Geometry check sheet. Reference: the model listing, model coordinates, mm. Round coordinates to 2 decimals unless told otherwise and drop trailing zeros. Order: outer loops, then holes, each group sorted by start corner. A loop starts at its lowest first (then second) coordinate and runs counter-clockwise, first axis right, second up. Notation, with made-up numbers: (86, 46) - (143, 46) arc R14 ccw to (143, 73) - close; hole circle Ø7 at (-33, 30.25). An arc over 180 degrees is marked (long way). Use a Markdown table: item, result. Add a question column.
(1) Thickness scan on line 1 along X through (y, z) = (-140, 2.2); line 2 along Y through (x, z) = (220, 1.35); line 3 along X through (y, z) = (100.5, 2.5). Record the ranges inside material, lowest first. Write a range as [from, to].
(2) Gauge pin test, flat end, axial feed: P1, Ø3, axis at x = 260, y = -100, coming from the +Z side. Record the tip position at first contact, or that the pin passes through.
(3) Section check B-B on y = -59.5. Record the boundary of the cut face in (x, z), then the cut area to 3 significant figures.
(4) Section check C-C on x = 17.5. Record the boundary of the cut face in (y, z).
(5) Section check A-A on z = 0.8. Give the number of separate pieces and of enclosed holes in the cut face, then the cut area to 3 significant figures.
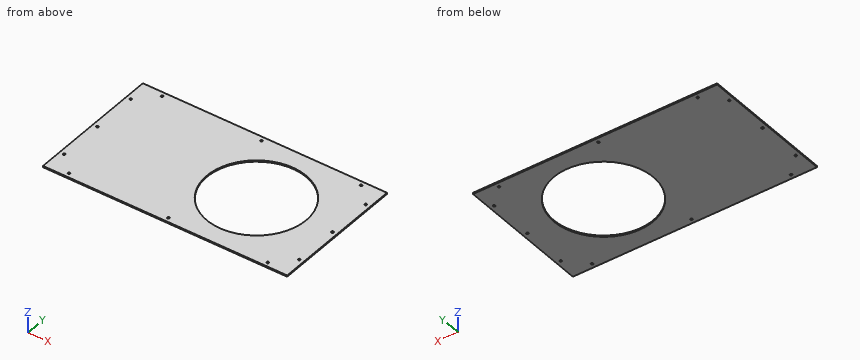
```python
from build123d import *

# Parameters (mm, degrees)
CROQUIS1_W              = 540
CROQUIS1_H              = 300
SALIENTE_EXTRUIR1_DEPTH = 3
CROQUIS2_R              = 2.5
CORTAR_EXTRUIR1_DEPTH   = 4
CROQUIS3_R              = 110
CORTAR_EXTRUIR2_DEPTH   = 4


with BuildPart() as part:
    # Croquis1 → Saliente-Extruir1 (new body)
    with BuildSketch(Plane.XY):
        Rectangle(CROQUIS1_W, CROQUIS1_H)
    extrude(amount=SALIENTE_EXTRUIR1_DEPTH)

    # Croquis2 → Cortar-Extruir1 (cut, through all)
    with BuildSketch(Plane.XY.offset(3)):
        with Locations((0, 140)):
            Circle(CROQUIS2_R)
        with Locations((-220, 140)):
            Circle(CROQUIS2_R)
        with Locations((-260, 0)):
            Circle(CROQUIS2_R)
        with Locations((-260, 100)):
            Circle(CROQUIS2_R)
        with Locations((-260, -100)):
            Circle(CROQUIS2_R)
        with Locations((220, 140)):
            Circle(CROQUIS2_R)
        with Locations((260, -100)):
            Circle(CROQUIS2_R)
        with Locations((260, 0)):
            Circle(CROQUIS2_R)
        with Locations((260, 100)):
            Circle(CROQUIS2_R)
        with Locations((220, -140)):
            Circle(CROQUIS2_R)
        with Locations((0, -140)):
            Circle(CROQUIS2_R)
        with Locations((-220, -140)):
            Circle(CROQUIS2_R)
    extrude(amount=-CORTAR_EXTRUIR1_DEPTH, mode=Mode.SUBTRACT)

    # Croquis3 → Cortar-Extruir2 (cut, through all)
    with BuildSketch(Plane.XY.offset(3)):
        with Locations((91.756190819, 0)):
            Circle(CROQUIS3_R)
    extrude(amount=-CORTAR_EXTRUIR2_DEPTH, mode=Mode.SUBTRACT)


solid = part.part
```
Check sheet entries:
| question | item | result |
|---|---|---|
| 1 | line 1 | x = [-270, -222.5], [-217.5, -2.5], [2.5, 217.5], [222.5, 270] |
| 1 | line 2 | y = [-150, -142.5], [-137.5, 137.5], [142.5, 150] |
| 1 | line 3 | x = [-270, -262.45], [-257.55, 47.04], [136.47, 257.55], [262.45, 270] |
| 2 | P1 | passes through |
| 3 | outline | (-270, 0) - (-0.76, 0) - (-0.76, 3) - (-270, 3) - close; (184.28, 0) - (270, 0) - (270, 3) - (184.28, 3) - close |
| 3 | area | 1,060 mm2 |
| 4 | outline | (-150, 0) - (-81.15, 0) - (-81.15, 3) - (-150, 3) - close; (81.15, 0) - (150, 0) - (150, 3) - (81.15, 3) - close |
| 5 | separate pieces | 1 |
| 5 | enclosed holes | 13 |
| 5 | area | 124,000 mm2 |
